```python
from build123d import *

# Parameters (mm, degrees)
BASEHEADSKE_R   = 18
BASEHEAD_DEPTH  = 24
CUTSOCKET_DEPTH = 12
FILLET_2_R      = 0.8


with BuildPart() as part:
    # BaseHeadSke → BaseHead (new body)
    with BuildSketch(Plane(origin=(0, 0, 0), x_dir=(0, 0, -1), z_dir=(1, 0, 0))):
        Circle(BASEHEADSKE_R)
    extrude(amount=BASEHEAD_DEPTH)

    # BodySke → BaseBody (revolve)
    with BuildSketch(Plane.XY, mode=Mode.PRIVATE) as basebody_sk:
        Polygon((0, 0), (124, 0), (124, 10.352), (122.352, 12), (0, 12), align=None)
    revolve(basebody_sk.sketch.rotate(Axis((0, 0, 0), (1, 0, 0)), 90), axis=Axis((0, 0, 0), (1, 0, 0)))

    # CutSocketSke → CutSocket (cut)
    with BuildSketch(Plane(origin=(0, 0, 0), x_dir=(0, 0, -1), z_dir=(1, 0, 0))):
        Polygon((0, 10.969655115), (-9.5, 5.484827557), (-9.5, -5.484827557), (0, -10.969655115), (9.5, -5.484827557), (9.5, 5.484827557), align=None)
    extrude(amount=CUTSOCKET_DEPTH, mode=Mode.SUBTRACT)

    # CutHoleSke → CutHole (revolve, cut)
    with BuildSketch(Plane.XY, mode=Mode.PRIVATE) as cuthole_sk:
        Polygon((0, 9.5), (13.6, 9.5), (19.084827557, 0), (0, 0), align=None)
    revolve(cuthole_sk.sketch.rotate(Axis((0, 0, 0), (1, 0, 0)), 90), axis=Axis((0, 0, 0), (1, 0, 0)), mode=Mode.SUBTRACT)

    # Fillet 2
    fillet_2_edges = [part.edges().sort_by_distance(p)[0] for p in [
        (0, 0, 18),
        (24, 0, 18),
        (24, 0, -12),
    ]]
    fillet(fillet_2_edges, radius=FILLET_2_R)


solid = part.part
```
Could you check a few things on this model? Use its own coordinates, in mm. A direction names the side the tool comes from. Give positions to 0.01 mm unless a question says otherwise; leave off trailing zeros. Loops run counter-clockwise (first coordinate to the right, second up) from the corner with the lowest first, then second, coordinate; pieces in that order, holes last. Notation, with made-up numbers: (3, -0.5) - (28, -0.5) arc R12 cw to (28, 5.5) - close; hole circle Ø7 at (13, 69.25). An arc over 180 degrees is marked (long way). Use one line per item in the form item = value.
1. Thinking about a two-plate mould opening in Y: for faces 1 (the face through (11.843, 17.847, 2.343)), 2 (the face through (5.916, -8.266, -4.684)), 3 (the face through (124, 0, 0)), which applies, released by +Y, released by -Y, zero draft, split by the parting line, or undercut?
Response values:
face_1 = split by the parting line
face_2 = undercut
face_3 = zero draft
2. I want a section at A-A (x = 65.5). Please give me the cut outline in (y, z), and give its area (3 significant figures).
Response values:
outline = circle Ø24 at (0, 0)
area = 452 mm²
3. On a 3-axis mill with a long thin cutter (end or side, diameter ignored), from which of +Z, -Z, +X, -X, +Y, -Y can I reach the whole of each face in a straight line? I mean faces 4 (the face through (24, 13, 0)), 5 (the face through (0, -7.4, -7.4)), 6 (the face through (5.9, 8.2, -4.8)). Say none if no direction works.
Response values:
face_4 = +X
face_5 = +Z, -Z, -X, +Y, -Y
face_6 = -X
4. I need wall thicknesses on probe 1 along Y at (x, z) = (13.2, 0); probe 2 along X at (y, z) = (-10, 13); probe 3 along Y at (x, z) = (46.5, -0.5). Which ranges of each line are inside material? Lowest first, please.
Response values:
probe_1 = -18 to -9.5, 9.5 to 18
probe_2 = 0 to 24
probe_3 = -11.99 to 11.99
5. I'm going to push flat-ended pins straight in: pin 1 Ø10 at (x, z) = (47.5, 0) entering from -Y; pin 2 Ø1.4 at (y, z) = (-6, -6) entering from -X; pin 3 Ø6 at (x, z) = (57, 12) entering from +Y. Where does each tip first touch, or does it pass through?
Response values:
pin_1 = -12
pin_2 = 13.78
pin_3 = 7.94
